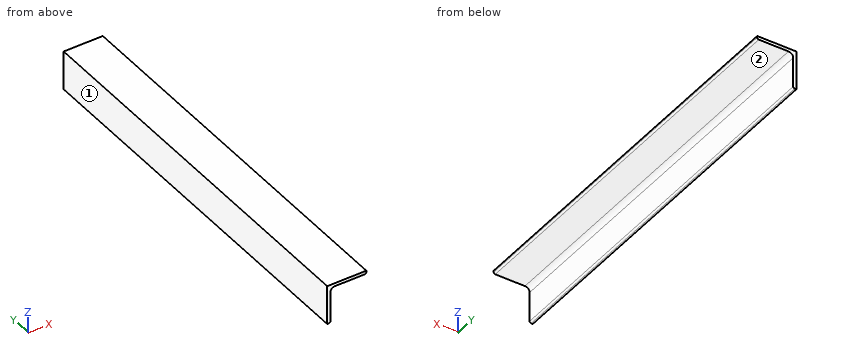
```python
from build123d import *

# Parameters (mm, degrees)
EXTRUDE_1_DEPTH = 758


with BuildPart() as part:
    # Эскиз1 → Бобышка-Вытянуть1 (new body)
    with BuildSketch(Plane(origin=(0, 0, 0), x_dir=(1, 0, 0), z_dir=(0, 1, 0))):
        with BuildLine():
            Line((0, 0), (0, 75))
            Line((0, 75), (3, 75))
            ThreePointArc((3, 75), (5.121320344, 74.121320344), (6, 72))
            Line((6, 72), (6, 15))
            ThreePointArc((6, 15), (8.636038969, 8.636038969), (15, 6))
            Line((15, 6), (72, 6))
            ThreePointArc((72, 6), (74.121320344, 5.121320344), (75, 3))
            Line((75, 3), (75, 0))
            Line((75, 0), (0, 0))
        make_face()
    extrude(amount=EXTRUDE_1_DEPTH)


solid = part.part
```
Check sheet for the modelled part. Datum: model origin and axes. Units: mm. Face numbers are marked on the shaded views. A direction names the side the tool comes from. Give positions to 0.01 mm unless a question says otherwise; leave off trailing zeros. Write each loop counter-clockwise with the first axis right and the second up, starting at its lowest first coordinate (ties: lowest second). Pieces come first, ordered by that corner, then holes. Notation, with made-up numbers: (43.5, 76) -> (53.5, 76) arc R32 cw to (53.5, 111) -> close; hole circle Ø11 at (-24, 30.25). An arc over 180 degrees is marked (long way). Use CSV: the item, a comma, the result in double quotes. Start each with the question number.
Q1. Cross-section at B-B on x = 55. Enter the section's corners in (y, z).
Q2. Tool access check on the marked faces 1 and 2. Record the directions out of +Z, -Z, +X, -X, +Y, -Y that give a thin tool (end or side, any length) a straight path to the whole face; none if there is none.
Q3. Depth check by flat-ended pin: P1, Ø10, axis at y = 332.5, z = -42, coming from the +X side. Enter the tip coordinate at first touch or a pass-through.
Q4. Cross-section at A-A on y = 549.5. Enter the section's corners in (x, z).
Q5. Scan lines: line 1 along Z through (x, y) = (33, 516); line 2 along X through (y, z) = (456.5, -32); line 3 along X through (y, z) = (462.5, -10). Record each from-to range of solid material in increasing order.
Q6. Cross-section at C-C on z = -33.5. Enter the section's corners in (x, y).
Working result:
1,outline,"(0, -6) -> (758, -6) -> (758, 0) -> (0, 0) -> close"
2,face 1,"+Z, -Z, -X, +Y, -Y"
2,face 2,"-Z, +X, +Y, -Y"
3,P1,"stops at x = 6"
4,outline,"(0, -75) -> (3, -75) arc R3 ccw to (6, -72) -> (6, -15) arc R9 cw to (15, -6) -> (72, -6) arc R3 ccw to (75, -3) -> (75, 0) -> (0, 0) -> close"
5,line 1,"z = -6 to 0"
5,line 2,"x = 0 to 6"
5,line 3,"x = 0 to 7.52"
6,outline,"(0, 0) -> (6, 0) -> (6, 758) -> (0, 758) -> close"
